Could you check a few things on this model? Use its own coordinates, in mm. A direction names the side the tool comes from. Round coordinates to 2 decimals unless told otherwise and drop trailing zeros. Loops run counter-clockwise (first coordinate to the right, second up) from the corner with the lowest first, then second, coordinate; pieces in that order, holes last. Notation, with made-up numbers: (1.25, 80) - (57.25, 80) arc R4 cw to (57.25, 85) - close; hole circle Ø1 at (-38, 5). An arc over 180 degrees is marked (long way). Use one line per item in the form item = value.
```python
from build123d import *

# Parameters (mm, degrees)
SKETCH1_R           = 7
BOSS_EXTRUDE1_DEPTH = 10
SKETCH2_W           = 10
SKETCH2_H           = 21
BOSS_EXTRUDE2_DEPTH = 2
SKETCH3_W           = 3.5
SKETCH3_H           = 8
BOSS_EXTRUDE3_DEPTH = 8
CUT_EXTRUDE1_DEPTH  = 27.172504657
SKETCH5_R           = 1.5
CUT_EXTRUDE2_DEPTH  = 27.172504657
CIRPATTERN1_COUNT   = 3


with BuildPart() as part:
    # Sketch1 → Boss-Extrude1 (new body)
    with BuildSketch(Plane(origin=(0, 0, 0), x_dir=(1, 0, 0), z_dir=(0, 1, 0))):
        with Locations(Location((0, 0, 0), (0, 0, 270))):
            Circle(SKETCH1_R)
    extrude(amount=BOSS_EXTRUDE1_DEPTH)

    # Sketch2 → Boss-Extrude2 (add)
    with BuildSketch(Plane.XZ):
        with Locations((0, 10.5)):
            Rectangle(SKETCH2_W, SKETCH2_H)
    boss_extrude2 = extrude(amount=-BOSS_EXTRUDE2_DEPTH)

    # Sketch3 → Boss-Extrude3 (add)
    with BuildSketch(Plane.XY.offset(21)):
        with Locations((-3.25, 6)):
            Rectangle(SKETCH3_W, SKETCH3_H)
        with Locations((3.25, 6)):
            Rectangle(SKETCH3_W, SKETCH3_H)
    boss_extrude3 = extrude(amount=-BOSS_EXTRUDE3_DEPTH)

    # Sketch4 → Cut-Extrude1 (cut, through all)
    with BuildSketch(Plane(origin=(5, 0, 0), x_dir=(0, 0, -1), z_dir=(1, 0, 0))):
        with BuildLine():
            Line((-21, 6), (-21, 11))
            Line((-21, 11), (-13, 11))
            Line((-13, 11), (-13, 6))
            ThreePointArc((-13, 6), (-17, 10), (-21, 6))
        make_face()
    cut_extrude1 = extrude(amount=-CUT_EXTRUDE1_DEPTH, mode=Mode.SUBTRACT)

    # Sketch5 → Cut-Extrude2 (cut, through all)
    with BuildSketch(Plane(origin=(5, 0, 0), x_dir=(0, 0, -1), z_dir=(1, 0, 0))):
        with Locations((-17, 6)):
            Circle(SKETCH5_R)
    cut_extrude2 = extrude(amount=-CUT_EXTRUDE2_DEPTH, mode=Mode.SUBTRACT)

    # CirPattern1: Boss-Extrude2, Boss-Extrude3, Cut-Extrude1, Cut-Extrude2 ×3 about axis
    cirpattern1_axis = Axis((0, 0, 0), (0, 1, 0))
    add([boss_extrude2.rotate(cirpattern1_axis, i * 360 / CIRPATTERN1_COUNT) for i in range(1, CIRPATTERN1_COUNT)])
    add([boss_extrude3.rotate(cirpattern1_axis, i * 360 / CIRPATTERN1_COUNT) for i in range(1, CIRPATTERN1_COUNT)])
    add([cut_extrude1.rotate(cirpattern1_axis, i * 360 / CIRPATTERN1_COUNT) for i in range(1, CIRPATTERN1_COUNT)], mode=Mode.SUBTRACT)
    add([cut_extrude2.rotate(cirpattern1_axis, i * 360 / CIRPATTERN1_COUNT) for i in range(1, CIRPATTERN1_COUNT)], mode=Mode.SUBTRACT)


solid = part.part
```
1. We'd pull the mould along Y, two halves only. Please class faces 6 (the face through (15.096, 6.451, -4.991)), 7 (the face through (-1.5, 4, 17)), 8 (the face through (10, 2, -6)): +Y half, -Y half, draft (parallel to the pull), parting line (faces both ways), or undercut.
Solution:
face_6 = undercut
face_7 = draft
face_8 = +Y half
2. If we section it at A-A, the plane z = 17: Write out the boundary of the cut face in (x, y), plus the area to 3 significant figures.
Solution:
outline = (-5, 0) - (5, 0) - (5, 4.5) - (1.5, 4.5) - (1.5, 2) - (-1.5, 2) - (-1.5, 4.5) - (-5, 4.5) - close; (-5, 7.5) - (-1.5, 7.5) - (-1.5, 10) - (-5, 10) - close; (1.5, 7.5) - (5, 7.5) - (5, 10) - (1.5, 10) - close
area = 55.0 mm^2
3. Please list where these lines run through material, in increasing order: line 1 along X through (y, z) = (8.5, 19); line 2 along X through (y, z) = (3.25, -4); line 3 along Y through (x, z) = (3, 17).
Solution:
line_1 = -5 to -1.5, 1.5 to 5
line_2 = -16.93 to -12.7, -5.74 to 5.74, 12.7 to 16.93
line_3 = 0 to 4.5, 7.5 to 10
4. If we section it at C-C, the plane x = 0: Write out the boundary of the cut face in (y, z).
Solution:
outline = (0, -7) - (10, -7) - (10, 7) - (2, 7) - (2, 21) - (0, 21) - close
5. If we section it at B-B, the plane y = 9.25: Write out the boundary of the cut face in (x, z), plus the area to 3 significant figures.
Solution:
outline = (-19.24, -5.34) - (-17.49, -8.37) - (-13.45, -6.04) - (-15.2, -3) - close; (-15.99, -10.96) - (-14.24, -14) - (-10.2, -11.66) - (-11.95, -8.63) - close; circle Ø14 at (0, 0); (-5, 14.67) - (-1.5, 14.67) - (-1.5, 19.33) - (-5, 19.33) - close; (1.5, 14.67) - (5, 14.67) - (5, 19.33) - (1.5, 19.33) - close; (10.2, -11.66) - (14.24, -14) - (15.99, -10.96) - (11.95, -8.63) - close; (13.45, -6.04) - (17.49, -8.37) - (19.24, -5.34) - (15.2, -3) - close
area = 252 mm^2
6. If we section it at D-D, the plane z = 0: Write out the boundary of the cut face in (x, y), plus the area to 3 significant figures.
Solution:
outline = (-10, 0) - (10, 0) - (10, 2) - (7, 2) - (7, 10) - (-7, 10) - (-7, 2) - (-10, 2) - close
area = 152 mm^2
7. For P1, Ø8, axis at x = 6.5, z = -3.5, coming from the +Y side; P2, Ø4, axis at y = 7.5, z = 17, coming from the -X side; P3, Ø1.5, axis at x = 12, y = 8, coming from the +Z side; P4, Ø6, axis at x = -13.5, z = 3, coming from the -Y side, each with a flat end and sliding along its axis, tell me the tip position at first contact or that it passes through.
Solution:
P1 = 10
P2 = -5
P3 = -4.78
P4 = through
8. On a 3-axis mill with a long thin cutter (end or side, diameter ignored), from which of +Z, -Z, +X, -X, +Y, -Y can I reach the whole of each face in a straight line? I mean faces 1 (the face through (-5, 4, 15)), 2 (the face through (5, 4, 15)), 3 (the face through (12.9, 4.03, -3.66)), 4 (the face through (-10, 2, -6)), 5 (the face through (-10.166, 3.819, -11.643)). Say none if no direction works.
Solution:
face_1 = +Z, -X, +Y, -Y
face_2 = +Z, +X, +Y, -Y
face_3 = +Z, +Y
face_4 = +Y
face_5 = -Z, +Y, -Y
